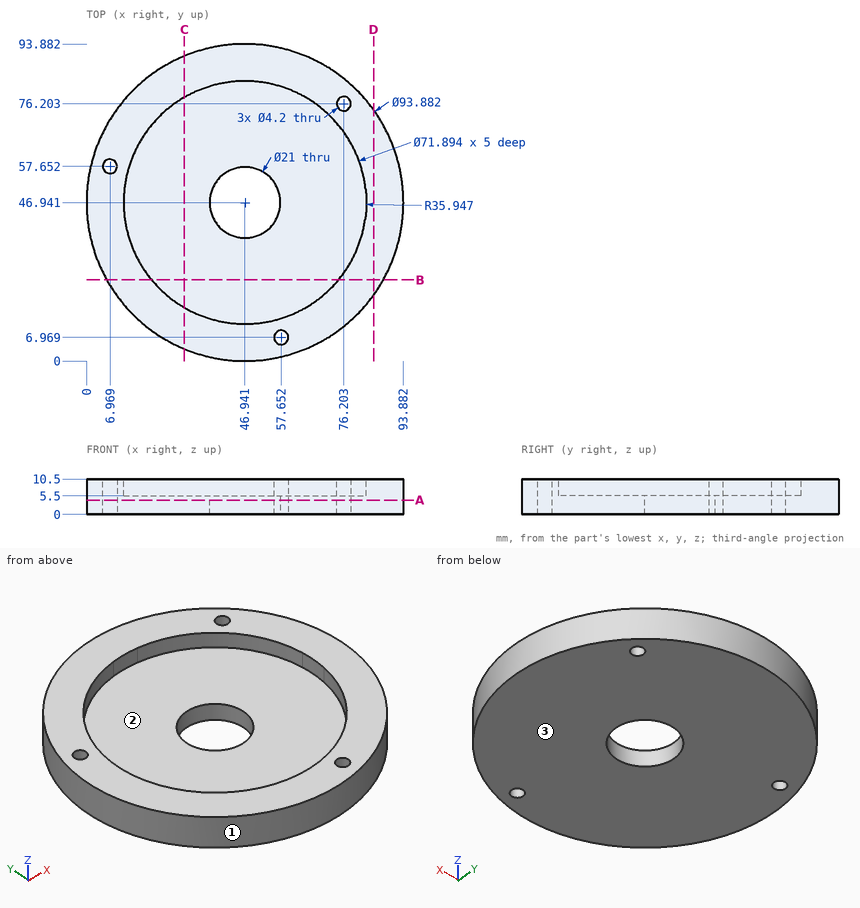
Job drawing, mm, ordinate dimensions from the low corner. One solid piece. Round coordinates to 2 decimals unless told otherwise and drop trailing zeros. Loops run counter-clockwise (first coordinate to the right, second up) from the corner with the lowest first, then second, coordinate; pieces in that order, holes last.
(1) Cut at B-B (y = 24). Give the cut face in (x, z) (1 decimal), plus the area to 3 significant figures.
(2) Cut at C-C (x = 29). Give the cut face in (y, z).
(3) Wall check: line 1 along X through (y, z) = (47.5, 1); line 2 along Y through (x, z) = (47, 8.25); line 3 along Y through (x, z) = (21.5, 9) (1 decimal). Give the ranges that are in metal, low to high.
(4) Drop flat-ended pins along their axis: pin 1 (6 mm diameter, centred on y = 32.5, z = 6, fed in from -X) (1 decimal); pin 2 (3.5 mm diameter, centred on x = 6.97, y = 57.65, fed in from -Z); pin 3 (5 mm diameter, centred on x = 26, z = 3, fed in from +Y); pin 4 (4 mm diameter, centred on x = 44.5, z = 6, fed in from -Y). Give the stop position or say it passes through.
(5) Cut at D-D (x = 85). Give the cut face in (y, z), plus the area to 3 significant figures.
(6) Cut at A-A (z = 4.25). Give the cut face in (x, y), plus the area to 3 significant figures.
(7) Two-plate mould, pull along X, no slides. Class the marked faces 1, 2 and 3: +X half, -X half, draft (parallel to the pull), parting line (faces both ways), or undercut.
Findings below:
1. outline: (6, 0) - (87.9, 0) - (87.9, 10.5) - (74.6, 10.5) - (74.6, 5.5) - (19.3, 5.5) - (19.3, 10.5) - (6, 10.5) - close
1. area: 583 mm2
2. outline: (3.56, 0) - (90.32, 0) - (90.32, 10.5) - (78.09, 10.5) - (78.09, 5.5) - (15.79, 5.5) - (15.79, 10.5) - (3.56, 10.5) - close
3. line 1: x = 0 to 36.46, 57.43 to 93.88
3. line 2: y = 0 to 10.99, 82.89 to 93.88
3. line 3: y = 7.5 to 21.5, 72.3 to 86.4
4. pin 1: stops at x = 1.4
4. pin 2: passes through
4. pin 3: stops at y = 90.11
4. pin 4: stops at y = 0
5. outline: (19.46, 0) - (74.42, 0) - (74.42, 10.5) - (19.46, 10.5) - close
5. area: 577 mm2
6. outline: circle Ø93.88 at (46.94, 46.94); hole circle Ø4.2 at (6.97, 57.65); hole circle Ø21 at (46.94, 46.94); hole circle Ø4.2 at (57.65, 6.97); hole circle Ø4.2 at (76.2, 76.2)
6. area: 6,530 mm2
7. face 1: parting line
7. face 2: undercut
7. face 3: draft
